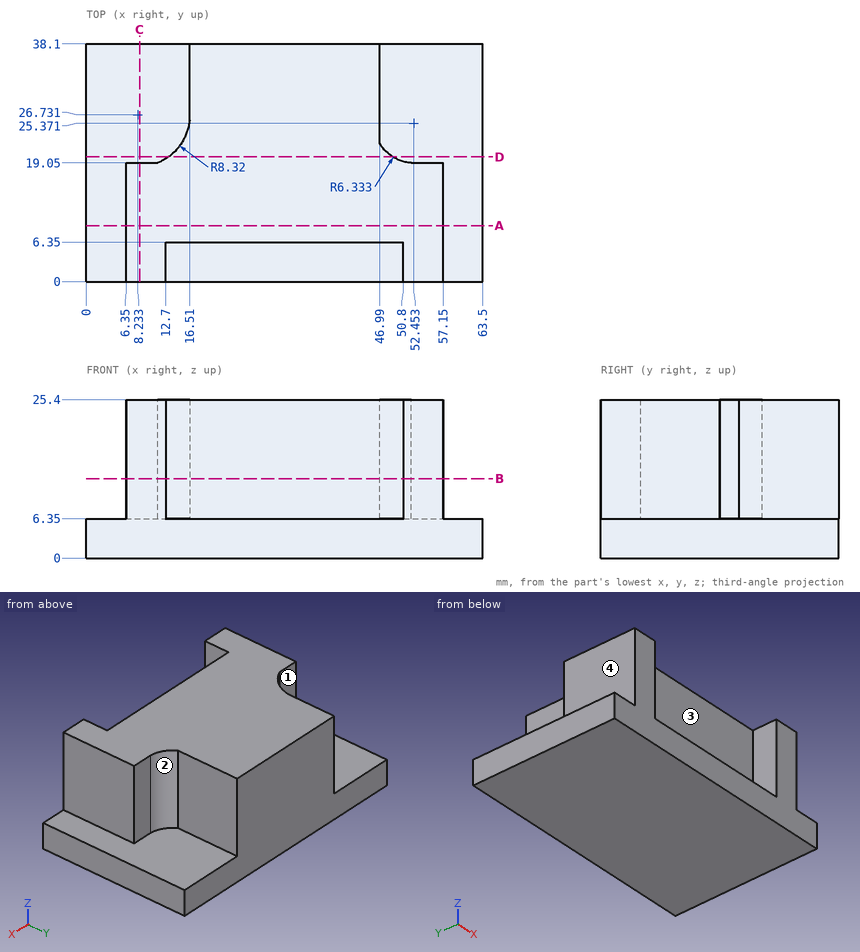
Geometry check sheet. Reference: drawing and pictorial views, mm from the part's lowest x, y, z. A direction names the side the tool comes from. Coordinates: 2 decimals unless noted, no trailing zeros. Loops run counter-clockwise (first coordinate to the right, second up) from the corner with the lowest first, then second, coordinate; pieces in that order, holes last. Notation, with made-up numbers: (-19.5, 46.5) - (-5.5, 46.5) arc R34 cw to (-5.5, 85.5) - close; hole circle Ø5 at (-31.75, 2.5). An arc over 180 degrees is marked (long way). Return JSON: item names as keys, results as strings.
1. Section check B-B, the plane z = 12.75. Record the boundary of the cut face in (x, y), then the cut area to 3 significant figures.
Established:
{"outline": "(6.35, 0) - (12.7, 0) - (12.7, 6.35) - (50.8, 6.35) - (50.8, 0) - (57.15, 0) - (57.15, 19.05) - (52.07, 19.05) arc R6.33 cw to (46.99, 22.17) - (46.99, 38.1) - (16.51, 38.1) - (16.51, 25.88) arc R8.32 cw to (11.43, 19.05) - (6.35, 19.05) - close", "area": "1,320 mm2"}
2. Tool access check on the marked faces 1, 2, 3 and 4. Record the directions out of +Z, -Z, +X, -X, +Y, -Y that give a thin tool (end or side, any length) a straight path to the whole face; none if there is none.
Established:
{"face 1": "+Z, -X, +Y", "face 2": "+Z, +X, +Y", "face 3": "+Z, -Y", "face 4": "+Z, -X, +Y, -Y"}
3. Thickness scan on L1, parallel to X at y = 2, z = 18; L2, parallel to X at y = 33, z = 19.5; L3, parallel to Z at x = 32, y = 4. Record the ranges inside material, lowest first.
Established:
{"L1": "x = 6.35 to 12.7, 50.8 to 57.15", "L2": "x = 16.51 to 46.99", "L3": "z = 0 to 6.35"}
4. Section check A-A, the plane y = 9. Record the boundary of the cut face in (x, z).
Established:
{"outline": "(0, 0) - (63.5, 0) - (63.5, 6.35) - (57.15, 6.35) - (57.15, 25.4) - (6.35, 25.4) - (6.35, 6.35) - (0, 6.35) - close"}
5. Section check C-C, the plane x = 8.5. Record the boundary of the cut face in (y, z), then the cut area to 3 significant figures.
Established:
{"outline": "(0, 0) - (38.1, 0) - (38.1, 6.35) - (19.05, 6.35) - (19.05, 25.4) - (0, 25.4) - close", "area": "605 mm2"}
6. Go/stop test with flat-tipped pins: pin 1 (5.5 mm diameter, centred on y = 12, z = 11.5, fed in from -X); pin 2 (2 mm diameter, centred on x = 43, z = 13.5, fed in from -Y); pin 3 (2 mm diameter, centred on x = 52, y = 13, fed in from -Z); pin 4 (5 mm diameter, centred on y = 2, z = 15.5, fed in from +X). Record where each tip stops, or that it passes through.
Established:
{"pin 1": "stops at x = 6.35", "pin 2": "stops at y = 6.35", "pin 3": "stops at z = 0", "pin 4": "stops at x = 57.15"}
7. Section check D-D, the plane y = 20. Record the boundary of the cut face in (x, z), then the cut area to 3 significant figures.
Established:
{"outline": "(0, 0) - (63.5, 0) - (63.5, 6.35) - (49.1, 6.35) - (49.1, 25.4) - (13.12, 25.4) - (13.12, 6.35) - (0, 6.35) - close", "area": "1,090 mm2"}
